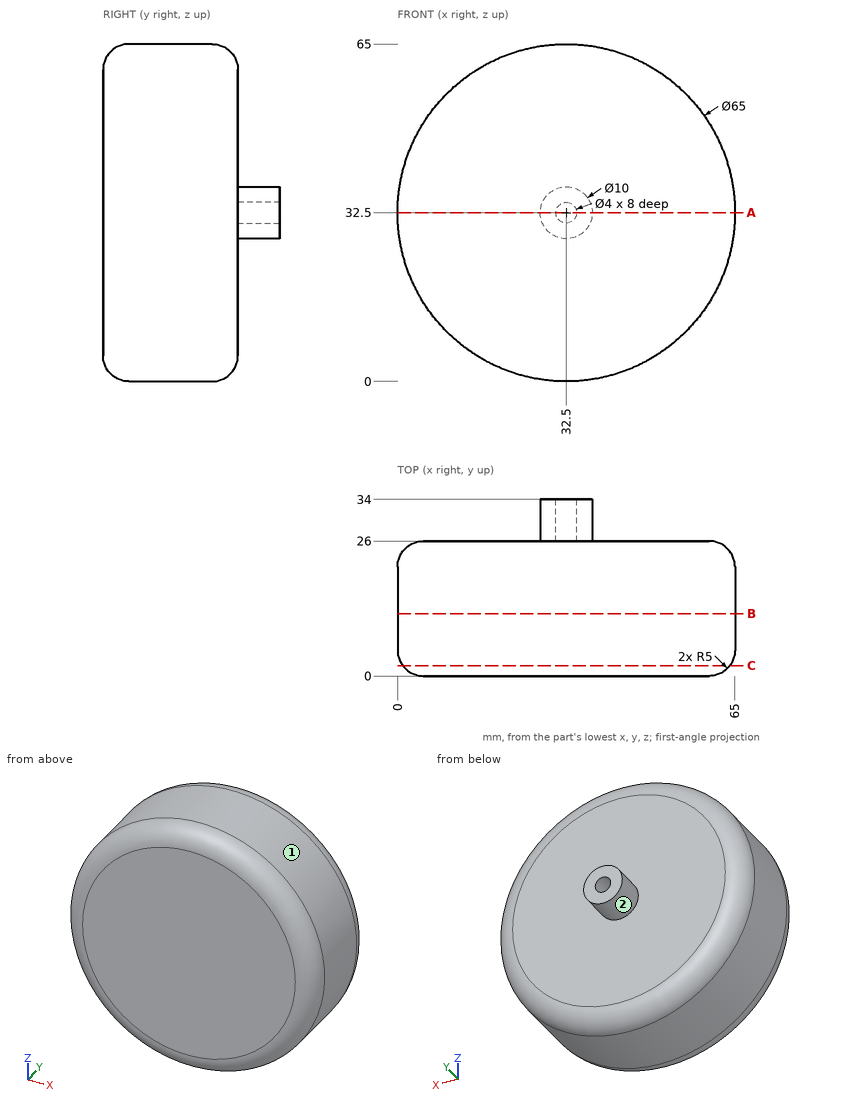
Geometry: see drawing. Coordinates: mm, zero at the bounding-box minimum. A direction names the side the tool comes from. Coordinates: 2 decimals unless noted, no trailing zeros. Loops run counter-clockwise (first coordinate to the right, second up) from the corner with the lowest first, then second, coordinate; pieces in that order, holes last. Notation, with made-up numbers: (38, -36) - (57, -36) arc R13 ccw to (57, -23) - close; hole circle Ø9 at (-25.5, 74.25). An arc over 180 degrees is marked (long way). Answer as CSV lines item,"result".
1. Section A-A (z = 32.5). Return loops of the section in (x, y), then the cut area to 3 significant figures.
Established:
outline,"(0, 5) arc R5 ccw to (5, 0) - (60, 0) arc R5 ccw to (65, 5) - (65, 21) arc R5 ccw to (60, 26) - (37.5, 26) - (37.5, 34) - (34.5, 34) - (34.5, 26) - (30.5, 26) - (30.5, 34) - (27.5, 34) - (27.5, 26) - (5, 26) arc R5 ccw to (0, 21) - close"
area,"1,720 mm2"
2. Contact query for flat-ended pins moving along their axis: pin 1 (5 mm diameter, centred on y = 7, z = 35, fed in from +X); pin 2 (1.5 mm diameter, centred on x = 54, y = 19.5, fed in from -Z); pin 3 (1.5 mm diameter, centred on x = 11.5, z = 40.5, fed in from +Y). Output: stop coordinate, or through.
Established:
pin 1,"stops at x = 65"
pin 2,"stops at z = 7.49"
pin 3,"stops at y = 26"
3. Section C-C (y = 2). Return loops of the section in (x, z), then the cut area to 3 significant figures.
Established:
outline,"circle Ø63 at (32.5, 32.5)"
area,"3,120 mm2"
4. Reachability of the marked faces 1 and 2 from +Z, -Z, +X, -X, +Y, -Y: full face, straight path, thin tool, end or side. Return the list, or none.
Established:
face 1,"+Y, -Y"
face 2,"+Y"
5. Ray query, line 1 (X direction, y = 29.25, z = 32.5); line 2 (Y direction, x = 46, z = 21); line 3 (Z direction, x = 32, y = 29). Return the intervals inside material, ascending.
Established:
line 1,"x = 27.5 to 30.5, 34.5 to 37.5"
line 2,"y = 0 to 26"
line 3,"z = 27.53 to 30.56, 34.44 to 37.47"
6. Section B-B (y = 12). Return loops of the section in (x, z).
Established:
outline,"circle Ø65 at (32.5, 32.5)"
